For this review, take the finished solid that the model builds, in its own axes (mm). Give positions to 0.01 mm unless a question says otherwise; leave off trailing zeros. Order: outer loops, then holes, each group sorted by start corner. A loop starts at its lowest first (then second) coordinate and runs counter-clockwise, first axis right, second up.
Item 1: Consider section B-B (y = -3). Give the boundary of the cut face in (x, z), plus the area to 3 significant figures.
Item 2: Consider section D-D (x = 1). Give the boundary of the cut face in (y, z), plus the area to 3 significant figures.
Item 3: For probe 1 along X at (y, z) = (-2, 0.3); probe 2 along Y at (x, z) = (-8.5, 0.45); probe 3 along X at (y, z) = (-2.75, 0.55), list the stretches that pass through material, from the lowest coordinate up.
Item 4: Consider section A-A (x = -10.5). Give the boundary of the cut face in (y, z).
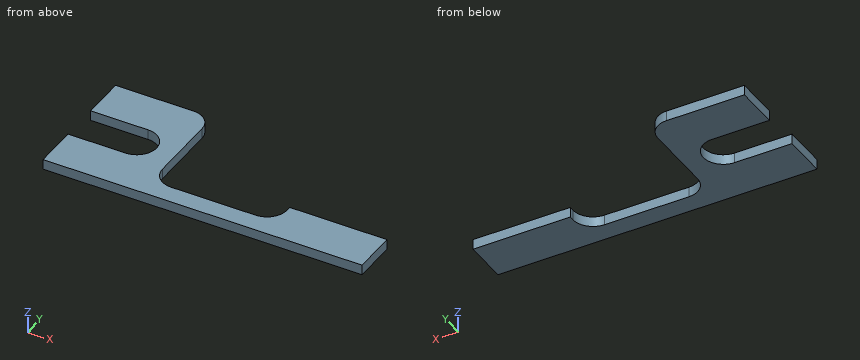
Autodesk Inventor part; units mm, degrees
ref_plane "Work Plane1" through (0, 0, 13.5128) normal (0, 0, 1) x (1, 0, 0)
ref_plane "YZ Plane" through (0, 0, 0) normal (1, 0, 0) x (0, 1, 0)
ref_plane "XZ Plane" through (0, 0, 0) normal (0, 1, 0) x (-1, 0, 0)
sketch "Sketch1" plane through (0, 0, 0) normal (0, 0, 1) x (1, 0, 0)
  line L0 (-12.7, 5.08) -> (12.7, 5.08)
  line L1 (12.7, 5.08) -> (12.7, -5.08)
  line L2 (12.7, -5.08) -> (-12.7, -5.08)
  line L3 (-12.7, -5.08) -> (-12.7, 5.08)
  point P0 (0, 0)
  point P1 (0, 5.08)
  point P2 (-12.7, 0)
  dimension "d0" = 25.4
  dimension "d1" = 10.16
extrude "Extrusion1" add sketch "Sketch1" along normal blind 0.8128
ref_plane "Work Plane1" through (0, 0, 13.5128) normal (0, 0, 1) x (1, 0, 0)
sketch "Sketch2" plane through (0, 0, 13.5128) normal (0, 0, 1) x (1, 0, 0)
  line L0 (12.7, 5.08) -> (12.7, -5.08)
  line L1 (-12.7, 5.08) -> (12.7, 5.08)
  line L2 (-12.7, -5.08) -> (-12.7, 5.08)
  line L3 (12.7, -5.08) -> (-12.7, -5.08)
  line L4 (-3.3655, 3.556) -> (3.3655, 3.556)
  line L5 (-3.3655, -3.556) -> (3.3655, -3.556)
  line L6 (-4.953, 1.9685) -> (-4.953, -1.9685)
  line L7 (4.953, 1.9685) -> (4.953, -1.9685)
  arc A0 (-3.3655, 3.556) -> (-4.953, 1.9685) centre (-3.3655, 1.9685) ccw
  arc A1 (-4.953, -1.9685) -> (-3.3655, -3.556) centre (-3.3655, -1.9685) ccw
  arc A2 (3.3655, -3.556) -> (4.953, -1.9685) centre (3.3655, -1.9685) ccw
  arc A3 (4.953, 1.9685) -> (3.3655, 3.556) centre (3.3655, 1.9685) ccw
  point P0 (0, 0)
  point P1 (0, 3.556)
  point P2 (0, -3.556)
  point P3 (-4.953, 0)
  point P4 (4.953, 0)
  dimension "d5" = 6.731
  dimension "d6" = 6.731
  dimension "d7" = 3.937
  dimension "d8" = 3.937
  dimension "d9" = 4.953
  dimension "d10" = 4.953
  dimension "d11" = 3.556
  dimension "d12" = 3.556
  dimension "d13" = 1.5875
  dimension "d14" = 1.5875
  dimension "d15" = 1.5875
  dimension "d16" = 1.5875
extrude "Extrusion2" cut sketch "Sketch2" against normal blind 25.4 contours L4 A3 L7 A2 L5 A1 L6 A0
sketch "Sketch3" plane through (0, 0, 13.5128) normal (0, 0, 1) x (1, 0, 0)
  arc A0 (-3.3655, 3.556) -> (-4.953, 1.9685) centre (-3.3655, 1.9685) ccw
  line L0 (-3.3655, 3.556) -> (3.3655, 3.556)
  arc A1 (4.953, 1.9685) -> (3.3655, 3.556) centre (3.3655, 1.9685) ccw
  line L1 (4.953, 1.9685) -> (4.953, -1.9685)
  arc A2 (3.3655, -3.556) -> (4.953, -1.9685) centre (3.3655, -1.9685) ccw
  line L2 (3.3655, -3.556) -> (-3.3655, -3.556)
  arc A3 (-4.953, -1.9685) -> (-3.3655, -3.556) centre (-3.3655, -1.9685) ccw
  line L3 (-4.953, -1.9685) -> (-4.953, 1.9685)
  line L4 (12.7, 5.08) -> (12.7, -5.08)
  line L5 (-12.7, 5.08) -> (12.7, 5.08)
  line L6 (-12.7, -5.08) -> (-12.7, 5.08)
  line L7 (12.7, -5.08) -> (-12.7, -5.08)
  line L8 (-12.7, 1.5875) -> (-8.128, 1.5875)
  line L9 (-12.7, -1.5875) -> (-8.128, -1.5875)
  arc A4 (-8.128, -1.5875) -> (-8.128, 1.5875) centre (-8.128, 0) ccw
  point P0 (0, 0)
  dimension "d19" = 4.572
  dimension "d20" = 3.4925
  dimension "d21" = 4.572
  dimension "d22" = 3.175
  dimension "d24" = 1.5875
extrude "Extrusion3" cut sketch "Sketch3" against normal blind 25.4 contours L8 A4 L9 L6
mirror "Mirror1" about plane through (0, 0, 0) normal (1, 0, 0) of "Extrusion3"
sketch "Sketch5" plane through (0, 0, 0.8128) normal (0, 0, 1) x (1, 0, 0)
  line L0 (4.953, 1.9685) -> (4.953, -1.9685) construction
  line L1 (-4.953, -1.9685) -> (4.953, -1.9685)
  line L2 (4.953, -1.9685) -> (4.953, 7.0011)
  line L3 (4.953, 7.0011) -> (-4.953, 7.0011)
  line L4 (-4.953, 7.0011) -> (-4.953, -1.9685)
  point P0 (0, 0)
extrude "Extrusion5" cut sketch "Sketch5" against normal blind 25.4
fillet "Fillet1" radius 1.524 2 edges at (-4.953, 5.08, 0.4064) (4.953, 5.08, 0.4064)
sketch "Sketch7" plane through (0, 0, 0.8128) normal (0, 0, 1) x (1, 0, 0)
  line L0 (8.128, -1.5875) -> (12.7, -1.5875) construction
  line L1 (12.7, -1.5875) -> (4.953, -1.5875)
  line L2 (4.953, -1.5875) -> (4.953, 5.08)
  line L3 (4.953, 5.08) -> (12.7, 5.08)
  line L4 (12.7, 5.08) -> (12.7, -1.5875)
  point P0 (0, 0)
extrude "Extrusion6" cut sketch "Sketch7" against normal through all
properties part number "headplate_largerCenter_frontsidecutout"
Resolved:
1. outline: (-12.7, 0) - (-4.57, 0) - (-4.57, 0.81) - (-12.7, 0.81) - close; (4.57, 0) - (12.7, 0) - (12.7, 0.81) - (4.57, 0.81) - close
1. area: 13.2 mm2
2. outline: (-5.08, 0) - (-3.56, 0) - (-3.56, 0.81) - (-5.08, 0.81) - close
2. area: 1.24 mm2
3. probe 1: x = -12.7 to -4.95, 4.95 to 12.7
3. probe 2: y = -5.08 to -1.59, 1.59 to 5.08
3. probe 3: x = -12.7 to -4.75, 4.75 to 12.7
4. outline: (-5.08, 0) - (-1.59, 0) - (-1.59, 0.81) - (-5.08, 0.81) - close; (1.59, 0) - (5.08, 0) - (5.08, 0.81) - (1.59, 0.81) - close
